Work out the finished part from the listing and answer in its coordinate system (mm). A direction names the side the tool comes from. Give positions to 0.01 mm unless a question says otherwise; leave off trailing zeros. Loops run counter-clockwise (first coordinate to the right, second up) from the corner with the lowest first, then second, coordinate; pieces in that order, holes last. Notation, with made-up numbers: (58.25, -36) - (113.25, -36) arc R29 ccw to (113.25, -15) - close; hole circle Ø6 at (14.25, -14). An arc over 180 degrees is marked (long way). One line per item, written item: value.
from build123d import *

# Parameters (mm, degrees)
SKETCH1_W                   = 300
SKETCH1_H                   = 300
SKETCH1_R                   = 70
SKETCH1_R_2                 = 65
SKETCH1_R_3                 = 62.5
SKETCH1_R_4                 = 55
SKETCH1_R_5                 = 20
SKETCH1_R_6                 = 17.5
BOSS_EXTRUDE1_DEPTH         = 10
SKETCH1_3_R                 = 65
SKETCH1_3_R_2               = 62.5
BOSS_EXTRUDE2_DEPTH         = 292
SKETCH1_4_R                 = 70
SKETCH1_4_R_2               = 65
BOSS_EXTRUDE3_DEPTH         = 422
SKETCH1_5_R                 = 20
SKETCH1_5_R_2               = 17.5
BOSS_EXTRUDE4_DEPTH         = 405
BOSS_EXTRUDE5_START         = -5
SKETCH3_R                   = 20
BOSS_EXTRUDE5_DEPTH         = 5
SKETCH4_R                   = 2.5
CUT_EXTRUDE1_DEPTH          = 5
BOSS_EXTRUDE6_DEPTH         = 427
RIB3_REACH                  = 474.318
SKETCH7_WALLS_W             = 1023.664705026
SKETCH7_WALLS_H             = 5
SKETCH7_WALLS_W_2           = 1024.247045089
SKETCH7_WALLS_W_3           = 5
SKETCH7_WALLS_H_2           = 1023.987417205
SKETCH7_WALLS_H_3           = 1024.344484495
M3_TAPPED_HOLE1_D           = 2.5
M3_TAPPED_HOLE1_DEPTH       = 7.5
M3_TAPPED_HOLE1_CSINK_D     = 3.05
M3_TAPPED_HOLE1_CSINK_ANGLE = 90
M3_TAPPED_HOLE1_TIP         = 0.751075774
SKETCH1_6_R                 = 62.5
SKETCH1_6_R_2               = 55
BOSS_EXTRUDE7_DEPTH         = 272


with BuildPart() as part:
    # Sketch1 → Boss-Extrude1 (new body)
    # profile 1 of 6: a face of its own
    with BuildSketch(Plane(origin=(0, 0, 0), x_dir=(1, 0, 0), z_dir=(0, 1, 0))):
        Rectangle(SKETCH1_W, SKETCH1_H)
        Circle(SKETCH1_R, mode=Mode.SUBTRACT)
    # profile 2 of 6: a face of its own
    with BuildSketch(Plane(origin=(0, 0, 0), x_dir=(1, 0, 0), z_dir=(0, 1, 0))):
        Circle(SKETCH1_R)
        Circle(SKETCH1_R_2, mode=Mode.SUBTRACT)
    # profile 3 of 6: a face of its own
    with BuildSketch(Plane(origin=(0, 0, 0), x_dir=(1, 0, 0), z_dir=(0, 1, 0))):
        Circle(SKETCH1_R_2)
        Circle(SKETCH1_R_3, mode=Mode.SUBTRACT)
    # profile 4 of 6: a face of its own
    with BuildSketch(Plane(origin=(0, 0, 0), x_dir=(1, 0, 0), z_dir=(0, 1, 0))):
        Circle(SKETCH1_R_3)
        Circle(SKETCH1_R_4, mode=Mode.SUBTRACT)
    # profile 5 of 6: a face of its own
    with BuildSketch(Plane(origin=(0, 0, 0), x_dir=(1, 0, 0), z_dir=(0, 1, 0))):
        Circle(SKETCH1_R_4)
        Circle(SKETCH1_R_5, mode=Mode.SUBTRACT)
    # profile 6 of 6: a face of its own
    with BuildSketch(Plane(origin=(0, 0, 0), x_dir=(1, 0, 0), z_dir=(0, 1, 0))):
        Circle(SKETCH1_R_5)
        with Locations(Location((0, 0, 0), (0, 0, 270))):
            Circle(SKETCH1_R_6, mode=Mode.SUBTRACT)
    extrude(amount=BOSS_EXTRUDE1_DEPTH)

    # Sketch1_3 → Boss-Extrude2 (add)
    with BuildSketch(Plane(origin=(0, 0, 0), x_dir=(1, 0, 0), z_dir=(0, 1, 0))):
        with Locations(Location((0, 0, 0), (0, 0, 270))):
            Circle(SKETCH1_3_R)
        with Locations(Location((0, 0, 0), (0, 0, 270))):
            Circle(SKETCH1_3_R_2, mode=Mode.SUBTRACT)
    extrude(amount=BOSS_EXTRUDE2_DEPTH)

    # Sketch1_4 → Boss-Extrude3 (add)
    with BuildSketch(Plane(origin=(0, 0, 0), x_dir=(1, 0, 0), z_dir=(0, 1, 0))):
        with Locations(Location((0, 0, 0), (0, 0, 270))):
            Circle(SKETCH1_4_R)
        with Locations(Location((0, 0, 0), (0, 0, 270))):
            Circle(SKETCH1_4_R_2, mode=Mode.SUBTRACT)
    extrude(amount=BOSS_EXTRUDE3_DEPTH)

    # Sketch1_5 → Boss-Extrude4 (add)
    with BuildSketch(Plane(origin=(0, 0, 0), x_dir=(1, 0, 0), z_dir=(0, 1, 0))):
        with Locations(Location((0, 0, 0), (0, 0, 270))):
            Circle(SKETCH1_5_R)
        with Locations(Location((0, 0, 0), (0, 0, 270))):
            Circle(SKETCH1_5_R_2, mode=Mode.SUBTRACT)
    extrude(amount=BOSS_EXTRUDE4_DEPTH)

    # Sketch3 → Boss-Extrude5 (add)
    with BuildSketch(Plane(origin=(0, 405, 0), x_dir=(1, 0, 0), z_dir=(0, 1, 0)).offset(BOSS_EXTRUDE5_START)):
        with Locations(Location((0, 0, 0), (0, 0, 270))):
            Circle(SKETCH3_R)
    extrude(amount=BOSS_EXTRUDE5_DEPTH)

    # Sketch4 → Cut-Extrude1 (cut)
    with BuildSketch(Plane(origin=(0, 405, 0), x_dir=(1, 0, 0), z_dir=(0, 1, 0))):
        with Locations(Location((0, 14.25, 0), (0, 0, 270))):
            Circle(SKETCH4_R)
        with Locations(Location((12.340862004, -7.125, 0), (0, 0, 270))):
            Circle(SKETCH4_R)
        with Locations(Location((-12.340862004, -7.125, 0), (0, 0, 270))):
            Circle(SKETCH4_R)
    extrude(amount=-CUT_EXTRUDE1_DEPTH, mode=Mode.SUBTRACT)

    # Sketch6 → Boss-Extrude6 (add)
    with BuildSketch(Plane(origin=(0, 0, 0), x_dir=(1, 0, 0), z_dir=(0, 1, 0))):
        Polygon((-120, 150), (120, 150), (150, 120), (150, -120), (120, -150), (-120, -150), (-150, -120), (-150, 120), align=None)
        Polygon((115, 145), (145, 115), (145, -115), (115, -145), (-115, -145), (-145, -115), (-145, 115), (-115, 145), align=None, mode=Mode.SUBTRACT)
    extrude(amount=BOSS_EXTRUDE6_DEPTH)

    # Sketch7 walls → Rib3 (add, up to next)
    with BuildSketch(Plane(origin=(0, 422, 0), x_dir=(1, 0, 0), z_dir=(0, 1, 0)), mode=Mode.PRIVATE) as rib3_sk1:
        with Locations((106.485337183, 0)):
            Rectangle(SKETCH7_WALLS_W, SKETCH7_WALLS_H)
    rib3_tool1 = extrude(rib3_sk1.sketch, amount=-RIB3_REACH, mode=Mode.PRIVATE) - part.part
    # Sketch7 walls → Rib3 (add, up to next)
    with BuildSketch(Plane(origin=(0, 422, 0), x_dir=(1, 0, 0), z_dir=(0, 1, 0)), mode=Mode.PRIVATE) as rib3_sk2:
        with Locations((-106.194167151, 0)):
            Rectangle(SKETCH7_WALLS_W_2, SKETCH7_WALLS_H)
    rib3_tool2 = extrude(rib3_sk2.sketch, amount=-RIB3_REACH, mode=Mode.PRIVATE) - part.part
    # Sketch7 walls → Rib3 (add, up to next)
    with BuildSketch(Plane(origin=(0, 422, 0), x_dir=(1, 0, 0), z_dir=(0, 1, 0)), mode=Mode.PRIVATE) as rib3_sk3:
        with Locations((0, 106.323981093)):
            Rectangle(SKETCH7_WALLS_W_3, SKETCH7_WALLS_H_2)
    rib3_tool3 = extrude(rib3_sk3.sketch, amount=-RIB3_REACH, mode=Mode.PRIVATE) - part.part
    # Sketch7 walls → Rib3 (add, up to next)
    with BuildSketch(Plane(origin=(0, 422, 0), x_dir=(1, 0, 0), z_dir=(0, 1, 0)), mode=Mode.PRIVATE) as rib3_sk4:
        with Locations((0, -106.145447448)):
            Rectangle(SKETCH7_WALLS_W_3, SKETCH7_WALLS_H_3)
    rib3_tool4 = extrude(rib3_sk4.sketch, amount=-RIB3_REACH, mode=Mode.PRIVATE) - part.part
    add(rib3_tool1.solids().sort_by_distance((106.485337183, 422, 0))[0])
    add(rib3_tool2.solids().sort_by_distance((-106.194167152, 422, 0))[0])
    add(rib3_tool3.solids().sort_by_distance((0, 422, -106.323981094))[0])
    add(rib3_tool4.solids().sort_by_distance((0, 422, 106.145447449))[0])

    # M3 Tapped Hole1
    with Locations(Plane(origin=(0, 422, 0), x_dir=(1, 0, 0), z_dir=(0, 1, 0))):
        with Locations((0, 130), (130, 0), (0, -130), (-130, 0)):
            CounterSinkHole(M3_TAPPED_HOLE1_D / 2, M3_TAPPED_HOLE1_CSINK_D / 2, depth=M3_TAPPED_HOLE1_DEPTH, counter_sink_angle=M3_TAPPED_HOLE1_CSINK_ANGLE)
            with Locations((0, 0, -(M3_TAPPED_HOLE1_DEPTH + M3_TAPPED_HOLE1_TIP / 2))):  # 118° drill point
                Cone(0, M3_TAPPED_HOLE1_D / 2, M3_TAPPED_HOLE1_TIP, mode=Mode.SUBTRACT)

    # Sketch1_6 → Boss-Extrude7 (add)
    with BuildSketch(Plane(origin=(0, 0, 0), x_dir=(1, 0, 0), z_dir=(0, 1, 0))):
        with Locations(Location((0, 0, 0), (0, 0, 270))):
            Circle(SKETCH1_6_R)
        with Locations(Location((0, 0, 0), (0, 0, 270))):
            Circle(SKETCH1_6_R_2, mode=Mode.SUBTRACT)
    extrude(amount=BOSS_EXTRUDE7_DEPTH)


solid = part.part
1. The mould has two halves that part along Z. Classify faces 1 (the cylindrical face through (-50.01, 213.12, 48.98)), 2 (the flat face through (150, 211, 2)), 3 (the flat face through (-2, 211, 150)): released by +Z, released by -Z, zero draft, split by the parting line, or undercut.
Output:
face 1: undercut
face 2: zero draft
face 3: released by +Z
2. Section B-B (x = 84.5) is taken. Write down the section's boundary in (y, z).
Output:
outline: (0, -150) - (427, -150) - (427, -145) - (10, -145) - (10, -2.5) - (422, -2.5) - (422, 2.5) - (10, 2.5) - (10, 145) - (427, 145) - (427, 150) - (0, 150) - close
3. For faces 4 (the flat face through (0, 405, 0)), 5 (the flat face through (-135, 216, 135)), 6 (the flat face through (-135, 216, -135)), 7 (the flat face through (135, 216, -135)), determine the directions among +Z, -Z, +X, -X, +Y, -Y from which every point of the face is accessible in a straight line to the end or side of a thin tool.
Output:
face 4: +Y
face 5: +Z, -X, +Y
face 6: -Z, -X, +Y
face 7: -Z, +X, +Y
4. Section C-C (z = 31) is taken. Write down the section's boundary in (x, y).
Output:
outline: (-150, 0) - (150, 0) - (150, 427) - (145, 427) - (145, 10) - (62.76, 10) - (62.76, 422) - (57.13, 422) - (57.13, 292) - (54.27, 292) - (54.27, 272) - (45.43, 272) - (45.43, 10) - (-45.43, 10) - (-45.43, 272) - (-54.27, 272) - (-54.27, 292) - (-57.13, 292) - (-57.13, 422) - (-62.76, 422) - (-62.76, 10) - (-145, 10) - (-145, 427) - (-150, 427) - close
5. Flat-ended cylindrical pins translate along their axes: pin 1 Ø1.5 at (x, z) = (0, 130) entering from +Y; pin 2 Ø6 at (x, z) = (-116.5, 44.5) entering from +Y; pin 3 Ø2 at (x, z) = (0, -130) entering from +Y. Find the tip coordinate at first contact, or state that the pin passes through.
Output:
pin 1: stops at y = 414.2
pin 2: stops at y = 10
pin 3: stops at y = 414.35
6. Section A-A (y = 208) is taken. Count the separate pieces of the cut face and the enclosed holes in it, and give its area (3 significant figures).
Output:
separate pieces: 2
enclosed holes: 6
area: 13,600 mm²
7. Find the intervals of material crossed by line 1 along Z through (x, y) = (73, 185); line 2 along X through (y, z) = (343, 0); line 3 along X through (y, z) = (262, 0), in increasing order.
Output:
line 1: z = -150 to -145, -2.5 to 2.5, 145 to 150
line 2: x = -150 to -65, -20 to -17.5, 17.5 to 20, 65 to 150
line 3: x = -150 to -55, -20 to -17.5, 17.5 to 20, 55 to 150
